Part model, mm, in its own coordinate system. Round coordinates to 2 decimals unless told otherwise and drop trailing zeros. Loops run counter-clockwise (first coordinate to the right, second up) from the corner with the lowest first, then second, coordinate; pieces in that order, holes last.
1) Band-saw the part on D-D, the plane x = -34.29. Write the cut outline in (y, z) (3 decimals), then the cut area to 3 significant figures.
2) Band-saw the part on C-C, the plane z = -29.21. Write the cut outline in (x, y) (3 decimals), then the cut area to 3 significant figures.
3) Band-saw the part on B-B, the plane x = -19.05. Write the cut outline in (y, z) (3 decimals), then the cut area to 3 significant figures.
4) Probe line 1 (X direction, y = 0.35, z = -3.81) (3 decimals); line 2 (Z direction, x = -34.29, y = 0.25) (3 decimals); line 3 (Z direction, x = -3, y = 0.15). List the from-to ranges inside material, lowest first.
5) Band-saw the part on A-A, the plane y = 0.45. Write the cut outline in (x, z) (3 decimals).
from build123d import *

# Parameters (mm, degrees)
SKETCH1_W           = 38.1
SKETCH1_H           = 33.02
BOSS_EXTRUDE1_DEPTH = 0.635
SKETCH2_R           = 1.905
CUT_EXTRUDE1_DEPTH  = 0.635
SKETCH3_R           = 6.35
CUT_EXTRUDE2_DEPTH  = 0.635


with BuildPart() as part:
    # Sketch1 → Boss-Extrude1 (new body)
    with BuildSketch(Plane(origin=(0, 0, 0), x_dir=(1, 0, 0), z_dir=(0, 1, 0))):
        with Locations((-19.05, 16.51)):
            Rectangle(SKETCH1_W, SKETCH1_H)
    extrude(amount=BOSS_EXTRUDE1_DEPTH)

    # Sketch2 → Cut-Extrude1 (cut)
    with BuildSketch(Plane(origin=(0, 0.635, 0), x_dir=(1, 0, 0), z_dir=(0, 1, 0))):
        with Locations((-34.29, 29.21)):
            Circle(SKETCH2_R)
        with Locations((-34.29, 3.81)):
            Circle(SKETCH2_R)
        with Locations((-3.81, 29.21)):
            Circle(SKETCH2_R)
        with Locations((-3.81, 3.81)):
            Circle(SKETCH2_R)
    extrude(amount=-CUT_EXTRUDE1_DEPTH, mode=Mode.SUBTRACT)

    # Sketch3 → Cut-Extrude2 (cut)
    with BuildSketch(Plane(origin=(0, 0.635, 0), x_dir=(1, 0, 0), z_dir=(0, 1, 0))):
        with Locations((-19.05, 16.51)):
            Circle(SKETCH3_R)
    extrude(amount=-CUT_EXTRUDE2_DEPTH, mode=Mode.SUBTRACT)


solid = part.part
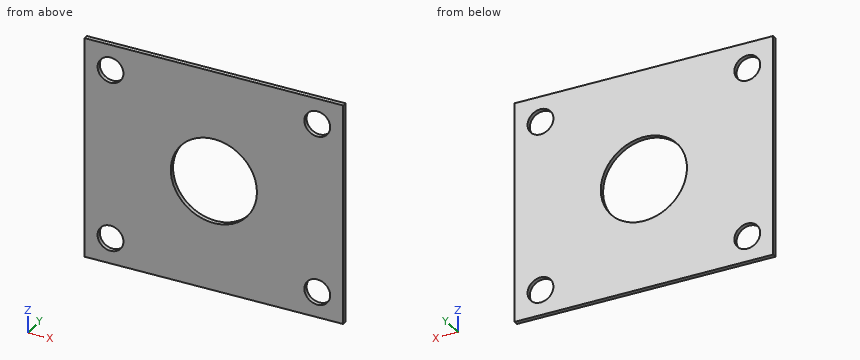
Reported:
1. outline: (0, -33.02) - (0.635, -33.02) - (0.635, -31.115) - (0, -31.115) - close; (0, -27.305) - (0.635, -27.305) - (0.635, -5.715) - (0, -5.715) - close; (0, -1.905) - (0.635, -1.905) - (0.635, 0) - (0, 0) - close
1. area: 16.1 mm2
2. outline: (-38.1, 0) - (-36.195, 0) - (-36.195, 0.635) - (-38.1, 0.635) - close; (-32.385, 0) - (-5.715, 0) - (-5.715, 0.635) - (-32.385, 0.635) - close; (-1.905, 0) - (0, 0) - (0, 0.635) - (-1.905, 0.635) - close
2. area: 19.4 mm2
3. outline: (0, -33.02) - (0.635, -33.02) - (0.635, -22.86) - (0, -22.86) - close; (0, -10.16) - (0.635, -10.16) - (0.635, 0) - (0, 0) - close
3. area: 12.9 mm2
4. line 1: x = -38.1 to -36.195, -32.385 to -5.715, -1.905 to 0
4. line 2: z = -33.02 to -31.115, -27.305 to -5.715, -1.905 to 0
4. line 3: z = -33.02 to -30.93, -27.49 to -5.53, -2.09 to 0
5. outline: (-38.1, -33.02) - (0, -33.02) - (0, 0) - (-38.1, 0) - close; hole circle Ø3.81 at (-34.29, -29.21); hole circle Ø3.81 at (-34.29, -3.81); hole circle Ø12.7 at (-19.05, -16.51); hole circle Ø3.81 at (-3.81, -29.21); hole circle Ø3.81 at (-3.81, -3.81)
